Answer from the drawing. Dimensions are ordinates in mm from the lowest x, y and z of the part. Give positions to 0.01 mm unless a question says otherwise; leave off trailing zeros. Write each loop counter-clockwise with the first axis right and the second up, starting at its lowest first coordinate (ties: lowest second). Pieces come first, ordered by that corner, then holes. Notation, with made-up numbers: M 49.5,15.25 L 61.5,15.25 A13 cw 61.5,35.25 Z; hole C 11,0 d4. An arc over 180 degrees is marked long. Put each result on its own line as item: value.
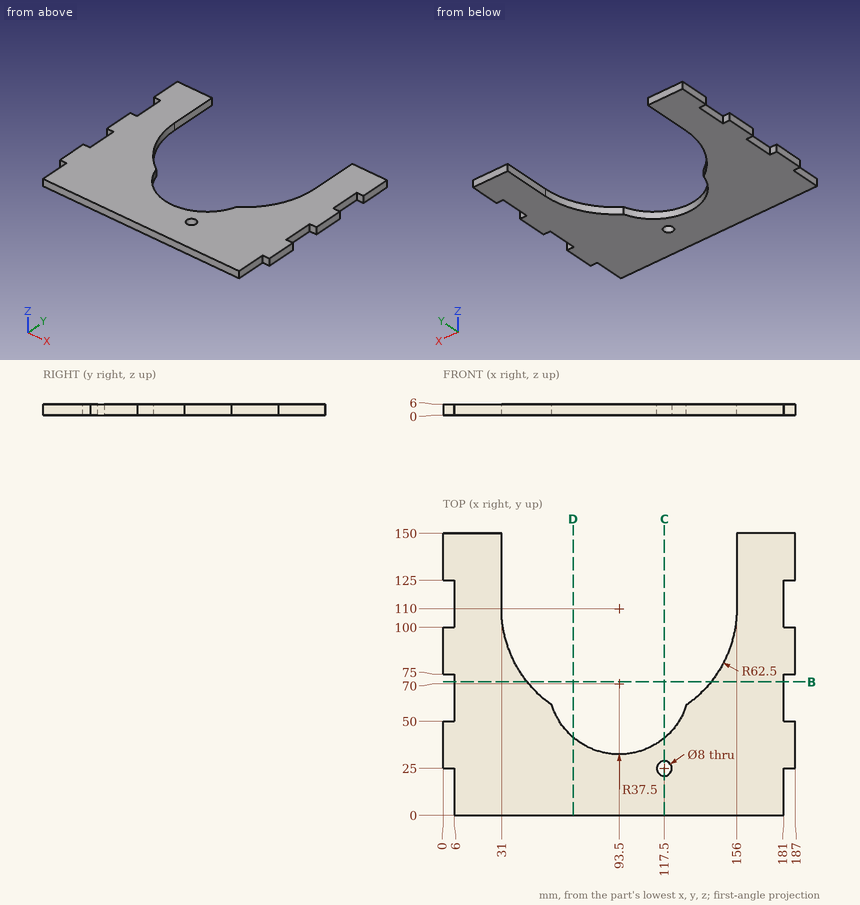
(1) Section C-C on x = 117.5 is taken. Determine the outline of the cut face in (y, z), and give its area (3 significant figures).
Result:
outline: M 0,0 L 21,0 L 21,6 L 0,6 Z; M 29,0 L 41.19,0 L 41.19,6 L 29,6 Z
area: 199 mm²
(2) Straight lines are drawn through the part: line 1 along X through (y, z) = (126, 5.55); line 2 along Y through (x, z) = (117.5, 3.35); line 3 along X through (y, z) = (38, 4.95). For each, find the intervals that lie inside material, in ascending order. Write a range as from..to.
Result:
line 1: x = 0..31, 156..187
line 2: y = 0..21, 29..41.19
line 3: x = 0..73.95, 113.05..187
(3) Given pin 1 Ø1.8 at (x, z) = (185, 2) entering from -Y; pin 2 Ø1 at (y, z) = (61, 1.5) entering from -X; pin 3 Ø1.8 at (y, z) = (10, 4.5) entering from +X, each flat-ended and moving along its own axis, determine where each tip first touches the part or whether it passes through.
Result:
pin 1: stops at y = 25
pin 2: stops at x = 6
pin 3: stops at x = 181
(4) Section B-B on y = 71 is taken. Determine the outline of the cut face in (x, z), and give its area (3 significant figures).
Result:
outline: M 6,0 L 44.66,0 L 44.66,6 L 6,6 Z; M 142.34,0 L 181,0 L 181,6 L 142.34,6 Z
area: 464 mm²
(5) Section D-D on x = 69 is taken. Determine the outline of the cut face in (y, z).
Result:
outline: M 0,0 L 41.61,0 L 41.61,6 L 0,6 Z
